For this review, use the dimensioned drawing (mm, ordinates from the lowest corner) and the shaded views. A direction names the side the tool comes from. Round coordinates to 2 decimals unless told otherwise and drop trailing zeros. Order: outer loops, then holes, each group sorted by start corner. A loop starts at its lowest first (then second) coordinate and runs counter-clockwise, first axis right, second up. Notation, with made-up numbers: M -21,34.25 L -8,34.25 A25 cw -8,68.25 Z; hole C 24.5,-34 d3. An arc over 180 degrees is marked long. Answer as CSV lines item,"result". Start each with the question number.
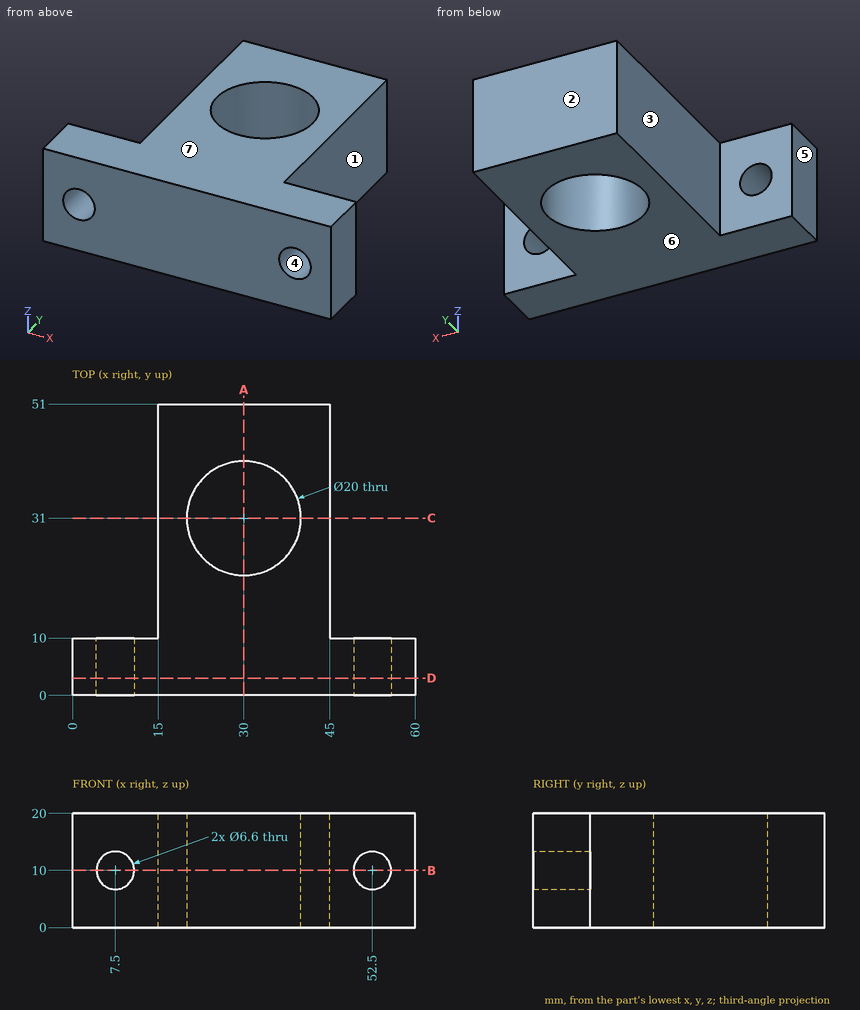
Item 1: Consider section A-A (x = 30). State the section outline as (y, z) points, and give its area (3 significant figures).
Item 2: Tool access review of the marked faces 1, 2 and 3: name each direction out of +Z, -Z, +X, -X, +Y, -Y from which nothing blocks a thin tool from reaching the whole face with its end or side.
Item 3: The part is to be moulded in two halves that separate along Z. For the marked faces 4, 5, 6 and 7, say which applies: +Z half, -Z half, draft (parallel to the pull), parting line (faces both ways), or undercut.
Item 4: Wall thickness on probe 1 along X at (y, z) = (6.5, 10); probe 2 along Y at (x, z) = (53, 18.25); probe 3 along Z at (x, y) = (51.5, 2.5): over which ranges is each line inside the solid? List them lowest first. Write a range as [from, to].
Item 5: Consider section D-D (y = 3). State the section outline as (x, z) points, and give its area (3 significant figures).
Item 6: For pin 1 (4 mm diameter, centred on x = 40, z = 2.5, fed in from -Y); pin 2 (7.5 mm diameter, centred on x = 56, z = 7, fed in from +Y); pin 3 (8 mm diameter, centred on y = 23, z = 5, fed in from -X); pin 4 (4 mm diameter, centred on y = 19, z = 12.5, fed in from +X), all flat-tipped, find the tip position at first contact; note any pin that passes through.
Item 7: Consider section B-B (z = 10). State the section outline as (x, y) points.
Item 8: Consider section C-C (y = 31). State the section outline as (x, z) points, and give its area (3 significant figures).
Reported:
1,outline,"M 0,0 L 21,0 L 21,20 L 0,20 Z; M 41,0 L 51,0 L 51,20 L 41,20 Z"
1,area,"620 mm²"
2,face 1,"+Z, -Z, +X, +Y"
2,face 2,"+Z, -Z, +X, -X, +Y"
2,face 3,"+Z, -Z, -X, +Y"
3,face 4,"undercut"
3,face 5,"draft"
3,face 6,"-Z half"
3,face 7,"+Z half"
4,probe 1,"x = [0, 4.2], [10.8, 49.2], [55.8, 60]"
4,probe 2,"y = [0, 10]"
4,probe 3,"z = [0, 6.86], [13.14, 20]"
5,outline,"M 0,0 L 60,0 L 60,20 L 0,20 Z; hole C 7.5,10 d6.6; hole C 52.5,10 d6.6"
5,area,"1,130 mm²"
6,pin 1,"stops at y = 0"
6,pin 2,"stops at y = 10"
6,pin 3,"stops at x = 15"
6,pin 4,"stops at x = 45"
7,outline,"M 0,0 L 4.2,0 L 4.2,10 L 0,10 Z; M 10.8,0 L 49.2,0 L 49.2,10 L 45,10 L 45,51 L 15,51 L 15,10 L 10.8,10 Z; M 55.8,0 L 60,0 L 60,10 L 55.8,10 Z; hole C 30,31 d20"
8,outline,"M 15,0 L 20,0 L 20,20 L 15,20 Z; M 40,0 L 45,0 L 45,20 L 40,20 Z"
8,area,"200 mm²"
